from build123d import *

# Parameters (mm, degrees)
BOSS_EXTRUDE1_DEPTH     = 9.525
SKETCH12_R              = 2.75
CUT_EXTRUDE2_DEPTH      = 278.704385318
CUT_EXTRUDE3_DEPTH      = 291.894698516
CUT_EXTRUDE3_DEPTH_BACK = 291.894698516
SKETCH13_R              = 2.75


with BuildPart() as part:
    # Sketch1 → Boss-Extrude1 (new, symmetric)
    with BuildSketch(Plane.XY):
        with BuildLine():
            Line((50, 0), (50, 243))
            ThreePointArc((50, 243), (41.213203436, 264.213203436), (20, 273))
            Line((20, 273), (-20, 273))
            ThreePointArc((-20, 273), (-41.213203436, 264.213203436), (-50, 243))
            Line((-50, 243), (-50, 0))
            Line((-50, 0), (-46.825, 0))
            Line((-46.825, 0), (-46.825, 243))
            ThreePointArc((-46.825, 243), (-38.968139405, 261.968139405), (-20, 269.825))
            Line((-20, 269.825), (20, 269.825))
            ThreePointArc((20, 269.825), (38.968139405, 261.968139405), (46.825, 243))
            Line((46.825, 243), (46.825, 0))
            Line((46.825, 0), (50, 0))
        make_face()
    extrude(amount=BOSS_EXTRUDE1_DEPTH, both=True)

    # Sketch12 → Cut-Extrude2 (cut, through all)
    with BuildSketch(Plane(origin=(0, 273, 0), x_dir=(1, 0, 0), z_dir=(0, 1, 0))):
        with Locations(Location((0, 0, 0), (0, 0, 270))):
            Circle(SKETCH12_R)
        with Locations(Location((-15, 0, 0), (0, 0, 270))):
            Circle(SKETCH12_R)
        with Locations(Location((15, 0, 0), (0, 0, 270))):
            Circle(SKETCH12_R)
    extrude(amount=-CUT_EXTRUDE2_DEPTH, mode=Mode.SUBTRACT)

    # Sketch13 → Cut-Extrude3 (cut, two sides: drawn at the far end of the back side and taken through both)
    with BuildSketch(Plane(origin=(50, 0, 0), x_dir=(0, 0, -1), z_dir=(1, 0, 0)).offset(-CUT_EXTRUDE3_DEPTH_BACK)):
        with Locations((0, 205)):
            Circle(SKETCH13_R)
        with Locations((0, 140)):
            Circle(SKETCH13_R)
        with Locations((0, 75)):
            Circle(SKETCH13_R)
    extrude(amount=CUT_EXTRUDE3_DEPTH + CUT_EXTRUDE3_DEPTH_BACK, mode=Mode.SUBTRACT)


solid = part.part
Verification items for the finished model (mm, model axes). A direction names the side the tool comes from. Coordinates: 2 decimals unless noted, no trailing zeros. Order: outer loops, then holes, each group sorted by start corner. A loop starts at its lowest first (then second) coordinate and runs counter-clockwise, first axis right, second up. Notation, with made-up numbers: M 20.5,35 L 70.5,35 A28 cw 70.5,64 Z; hole C 36.5,42.25 d1. An arc over 180 degrees is marked long. One line per item, written item: value. Start each with the question number.
Item 1: Mould release check, pull along X, two halves, no side actions. Record for faces 3 (the cylindrical face through (-48.435, 77.727, 0.358)), 4 (the flat face through (46.825, 123, 0)), 5 (the cylindrical face through (41.445, 263.979, 0.133)): released by +X, released by -X, zero draft, split by the parting line, or undercut.
Item 2: Scan lines: probe 1 along X at (y, z) = (139.5, 3.75) (3 decimals); probe 2 along Z at (x, y) = (48, 75) (3 decimals); probe 3 along Y at (x, z) = (-8.5, -0.5) (3 decimals). Record each from-to range of solid material in increasing order.
Item 3: Gauge pin test, flat end, axial feed: pin 1 (6.5 mm diameter, centred on x = 0, z = 0, fed in from -Y) (3 decimals). Record the tip position at first contact, or that the pin passes through.
Item 4: Sectioned sample at D-D (z = -5.5). Enter the section's corners in (x, y) (3 decimals), then the cut area to 3 significant figures.
Item 5: Access from +Z, -Z, +X, -X, +Y, -Y to the whole of each face (thin tool, end or side, straight path). Record for faces 1 (the cylindrical face through (48.39, 137.315, 0.596)), 2 (the cylindrical face through (-39.176, 261.758, 0.133)).
Item 6: Sectioned sample at B-B (x = 0). Enter the section's corners in (y, z) (3 decimals).
Item 7: Sectioned sample at A-A (y = 140). Enter the section's corners in (x, z) (3 decimals).
Item 8: Sectioned sample at C-C (y = 236). Enter the section's corners in (x, z) (3 decimals), then the cut area to 3 significant figures.
Conclusion:
1. face 3: zero draft
1. face 4: undercut
1. face 5: released by +X
2. probe 1: x = -50 to -46.825, 46.825 to 50
2. probe 2: z = -9.525 to -2.75, 2.75 to 9.525
2. probe 3: y = 269.825 to 273
3. pin 1: stops at y = 269.825
4. outline: M -50,0 L -46.825,0 L -46.825,243 A26.825 cw -20,269.825 L 20,269.825 A26.825 cw 46.825,243 L 46.825,0 L 50,0 L 50,243 A30 ccw 20,273 L -20,273 A30 ccw -50,243 Z
4. area: 1,950 mm^2
5. face 1: +X, -X
5. face 2: +Z, -Z, -Y
6. outline: M 269.825,-9.525 L 273,-9.525 L 273,-2.75 L 269.825,-2.75 Z; M 269.825,2.75 L 273,2.75 L 273,9.525 L 269.825,9.525 Z
7. outline: M -50,-9.525 L -46.825,-9.525 L -46.825,-2.75 L -50,-2.75 Z; M -50,2.75 L -46.825,2.75 L -46.825,9.525 L -50,9.525 Z; M 46.825,-9.525 L 50,-9.525 L 50,-2.75 L 46.825,-2.75 Z; M 46.825,2.75 L 50,2.75 L 50,9.525 L 46.825,9.525 Z
8. outline: M -50,-9.525 L -46.825,-9.525 L -46.825,9.525 L -50,9.525 Z; M 46.825,-9.525 L 50,-9.525 L 50,9.525 L 46.825,9.525 Z
8. area: 121 mm^2
